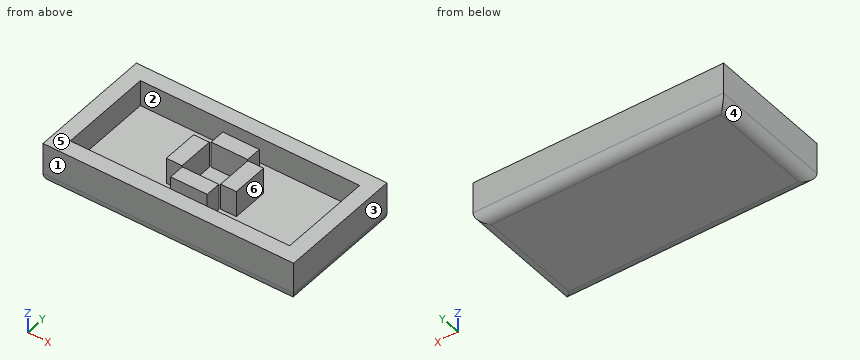
from build123d import *

# Parameters (mm, degrees)
SKETCH_W      = 24
SKETCH_H      = 12
PAD_DEPTH     = 1.5
SKETCH002_W   = 3.5
SKETCH002_H   = 1.5
SKETCH002_W_2 = 1.5
SKETCH002_H_2 = 3.5
PAD002_DEPTH  = 4
SKETCH003_W   = 24
SKETCH003_H   = 12
SKETCH003_W_2 = 21
SKETCH003_H_2 = 9
PAD003_DEPTH  = 4
FILLET_R      = 1


with BuildPart() as part:
    # Sketch → Pad (new body)
    with BuildSketch(Plane.XY):
        Rectangle(SKETCH_W, SKETCH_H)
    extrude(amount=PAD_DEPTH)

    # Sketch002 → Pad002 (join)
    with BuildSketch(Plane.XY):
        with Locations((0, 2.6)):
            Rectangle(SKETCH002_W, SKETCH002_H)
        with Locations((0, -2.6)):
            Rectangle(SKETCH002_W, SKETCH002_H)
        with Locations((-2.6, 0)):
            Rectangle(SKETCH002_W_2, SKETCH002_H_2)
        with Locations((2.6, 0)):
            Rectangle(SKETCH002_W_2, SKETCH002_H_2)
    extrude(amount=PAD002_DEPTH)

    # Sketch003 → Pad003 (join)
    with BuildSketch(Plane.XY):
        Rectangle(SKETCH003_W, SKETCH003_H)
        Rectangle(SKETCH003_W_2, SKETCH003_H_2, mode=Mode.SUBTRACT)
    extrude(amount=PAD003_DEPTH)

    # Fillet
    fillet_edges = [part.edges().sort_by_distance(p)[0] for p in [
        (-12, 0, 0),
        (0, -6, 0),
        (12, 0, 0),
        (0, 6, 0),
    ]]
    fillet(fillet_edges, radius=FILLET_R)


solid = part.part
Geometry: final body of the model. Coordinates: model frame, mm. Face numbers are marked on the shaded views. A direction names the side the tool comes from. Coordinates: 2 decimals unless noted, no trailing zeros. Order: outer loops, then holes, each group sorted by start corner. A loop starts at its lowest first (then second) coordinate and runs counter-clockwise, first axis right, second up.
1) Section D-D (x = 4.5). Return loops of the section in (y, z).
Result sheet:
outline: (-6, 1) arc R1 ccw to (-5, 0) - (5, 0) arc R1 ccw to (6, 1) - (6, 4) - (4.5, 4) - (4.5, 1.5) - (-4.5, 1.5) - (-4.5, 4) - (-6, 4) - close
2) Set-up query: the marked faces 1 and 2. Return all of +Z, -Z, +X, -X, +Y, -Y with unobstructed straight access to the full face (end or side cutting, diameter ignored); none if empty.
Result sheet:
face 1: +Z, -Z, +X, -X, -Y
face 2: +Z
3) First-contact query: P1, Ø1, axis at x = -8, y = 3, coming from the +Z side. Flat tip, straight axial feed; report the tip coordinate or a pass-through.
Result sheet:
P1: stops at z = 1.5
4) Section C-C (y = 0.75). Return loops of the section in (x, z).
Result sheet:
outline: (-12, 1) arc R1 ccw to (-11, 0) - (11, 0) arc R1 ccw to (12, 1) - (12, 4) - (10.5, 4) - (10.5, 1.5) - (3.35, 1.5) - (3.35, 4) - (1.85, 4) - (1.85, 1.5) - (-1.85, 1.5) - (-1.85, 4) - (-3.35, 4) - (-3.35, 1.5) - (-10.5, 1.5) - (-10.5, 4) - (-12, 4) - close
5) Draft query along X for the marked faces 3, 4, 5 and 6. Return one class per face: released by +X, released by -X, zero draft, split by the parting line, or undercut.
Result sheet:
face 3: released by +X
face 4: released by -X
face 5: zero draft
face 6: undercut
6) Section B-B (x = 0.25). Return loops of the section in (y, z), then the cut area to 3 significant figures.
Result sheet:
outline: (-6, 1) arc R1 ccw to (-5, 0) - (5, 0) arc R1 ccw to (6, 1) - (6, 4) - (4.5, 4) - (4.5, 1.5) - (3.35, 1.5) - (3.35, 4) - (1.85, 4) - (1.85, 1.5) - (-1.85, 1.5) - (-1.85, 4) - (-3.35, 4) - (-3.35, 1.5) - (-4.5, 1.5) - (-4.5, 4) - (-6, 4) - close
area: 32.6 mm2
7) Section A-A (z = 2.5). Return loops of the section in (x, y), then the cut area to 3 significant figures.
Result sheet:
outline: (-12, -6) - (12, -6) - (12, 6) - (-12, 6) - close; (-3.35, -1.75) - (-1.85, -1.75) - (-1.85, 1.75) - (-3.35, 1.75) - close; (-1.75, -3.35) - (1.75, -3.35) - (1.75, -1.85) - (-1.75, -1.85) - close; (-1.75, 1.85) - (1.75, 1.85) - (1.75, 3.35) - (-1.75, 3.35) - close; (1.85, -1.75) - (3.35, -1.75) - (3.35, 1.75) - (1.85, 1.75) - close; hole (-10.5, -4.5) - (10.5, -4.5) - (10.5, 4.5) - (-10.5, 4.5) - close
area: 120 mm2
8) Ray query, probe 1 along X at (y, z) = (-0.25, 2.25); probe 2 along Y at (x, z) = (0, 1.9); probe 3 along X at (y, z) = (3.25, 2.55). Return the intervals inside material, ascending.
Result sheet:
probe 1: x = -12 to -10.5, -3.35 to -1.85, 1.85 to 3.35, 10.5 to 12
probe 2: y = -6 to -4.5, -3.35 to -1.85, 1.85 to 3.35, 4.5 to 6
probe 3: x = -12 to -10.5, -1.75 to 1.75, 10.5 to 12
